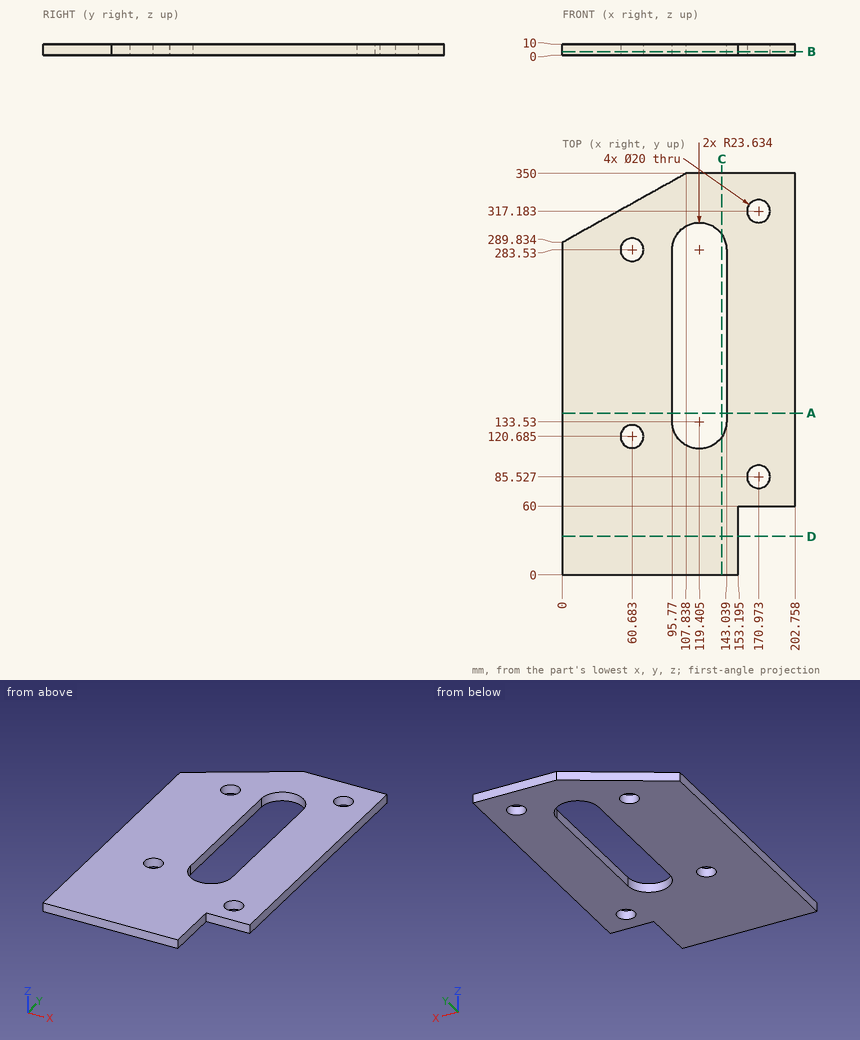
Can you work these out from the drawing? Everything is in mm from the part's minimum corner. Give positions to 0.01 mm unless a question says otherwise; leave off trailing zeros. Loops run counter-clockwise (first coordinate to the right, second up) from the corner with the lowest first, then second, coordinate; pieces in that order, holes last. Notation, with made-up numbers: (41, 68.5) -> (97, 68.5) arc R25 ccw to (97, 104.5) -> close; hole circle Ø3 at (50, -19.75). An arc over 180 degrees is marked (long way). Put each result on its own line as item: value.
(1) Imagine slicing it at A-A on y = 141. Write out the boundary of the cut face in (x, z).
Computed:
outline: (0, 0) -> (95.77, 0) -> (95.77, 10) -> (0, 10) -> close; (143.04, 0) -> (202.76, 0) -> (202.76, 10) -> (143.04, 10) -> close
(2) Imagine slicing it at B-B on z = 3.25. Write out the boundary of the cut face in (x, y) (1 decimal), plus the area to 3 significant figures.
Computed:
outline: (0, 0) -> (153.2, 0) -> (153.2, 60) -> (202.8, 60) -> (202.8, 350) -> (107.8, 350) -> (0, 289.8) -> close; hole circle Ø20 at (60.7, 120.7); hole circle Ø20 at (60.7, 283.5); hole (95.8, 133.5) arc R23.6 ccw to (143, 133.5) -> (143, 283.5) arc R23.6 ccw to (95.8, 283.5) -> close; hole circle Ø20 at (171, 85.5); hole circle Ø20 at (171, 317.2)
area: 54,600 mm^2
(3) Imagine slicing it at C-C on x = 139. Write out the boundary of the cut face in (y, z) (1 decimal), plus the area to 3 significant figures.
Computed:
outline: (0, 0) -> (120.3, 0) -> (120.3, 10) -> (0, 10) -> close; (296.7, 0) -> (350, 0) -> (350, 10) -> (296.7, 10) -> close
area: 1,740 mm^2
(4) I'm going to push flat-ended pins straight in: pin 1 Ø6 at (y, z) = (234, 1) entering from -X; pin 2 Ø1 at (y, z) = (44, 8.5) entering from +X (1 decimal); pin 3 Ø16 at (x, y) = (170.97, 317.18) entering from -Z. Where does each tip first touch, or does it pass through?
Computed:
pin 1: x = 0
pin 2: x = 153.2
pin 3: through
(5) Please list where these lines run through material, in increasing order: probe 1 along X at (y, z) = (182.5, 5.25); probe 2 along X at (y, z) = (50, 4.25) (1 decimal); probe 3 along Y at (x, z) = (123.5, 3.5). Write a range as [from, to].
Computed:
probe 1: [0, 95.77], [143.04, 202.76]
probe 2: [0, 153.2]
probe 3: [0, 110.25], [306.81, 350]
(6) Imagine slicing it at D-D on y = 33.5. Write out the boundary of the cut face in (x, z) (1 decimal), plus the area to 3 significant figures.
Computed:
outline: (0, 0) -> (153.2, 0) -> (153.2, 10) -> (0, 10) -> close
area: 1,530 mm^2
